from build123d import *

# Parameters (mm, degrees)
BOSS_EXTRUDE1_DEPTH = 19.05
SKETCH2_W           = 25.4
SKETCH2_H           = 6.35
BOSS_EXTRUDE2_DEPTH = 38.1
SKETCH3_R           = 6.35
CUT_EXTRUDE1_DEPTH  = 172.685024099
FILLET1_R           = 6.35
FILLET2_R           = 2.54
FILLET3_R           = 2.54


with BuildPart() as part:
    # Sketch1 → Boss-Extrude1 (new body)
    with BuildSketch(Plane(origin=(0, 0, 0), x_dir=(1, 0, 0), z_dir=(0, 1, 0))):
        with BuildLine():
            Line((-94.376875, 43.859194763), (4.54025, 27.568636708))
            ThreePointArc((4.54025, 27.568636708), (27.94, 0), (4.54025, -27.568636708))
            Line((4.54025, -27.568636708), (-94.376875, -43.859194763))
            ThreePointArc((-94.376875, -43.859194763), (-146.05, 0), (-94.376875, 43.859194763))
        make_face()
    extrude(amount=BOSS_EXTRUDE1_DEPTH)

    # Sketch2 → Boss-Extrude2 (add)
    with BuildSketch(Plane(origin=(0, 19.05, 0), x_dir=(1, 0, 0), z_dir=(0, 1, 0))):
        with Locations((-101.6, 22.225)):
            Rectangle(SKETCH2_W, SKETCH2_H)
        with Locations((-101.6, -22.225)):
            Rectangle(SKETCH2_W, SKETCH2_H)
    extrude(amount=BOSS_EXTRUDE2_DEPTH)

    # Sketch3 → Cut-Extrude1 (cut, through all)
    with BuildSketch(Plane.XY.offset(25.4)):
        with BuildLine():
            Line((-114.3, 57.15), (-114.3, 34.925))
            ThreePointArc((-114.3, 34.925), (-101.6, 47.625), (-88.9, 34.925))
            Line((-88.9, 34.925), (-88.9, 57.15))
            Line((-88.9, 57.15), (-114.3, 57.15))
        make_face()
        with Locations((-101.6, 34.925)):
            Circle(SKETCH3_R)
    extrude(amount=-CUT_EXTRUDE1_DEPTH, mode=Mode.SUBTRACT)

    # Fillet1
    fillet1_edges = [part.edges().sort_by_distance(p)[0] for p in [
        (27.94, 19.05, 0),
        (-44.9183125, 19.05, -35.713915735),
        (-146.05, 19.05, 0),
        (-44.9183125, 19.05, 35.713915735),
    ]]
    fillet(fillet1_edges, radius=FILLET1_R)

    # Fillet2
    fillet2_edges = [part.edges().sort_by_distance(p)[0] for p in [
        (-44.9183125, 0, -35.713915735),
        (27.94, 0, 0),
        (-44.9183125, 0, 35.713915735),
        (-146.05, 0, 0),
    ]]
    fillet(fillet2_edges, radius=FILLET2_R)

    # Fillet3
    fillet3_edges = [part.edges().sort_by_distance(p)[0] for p in [
        (-88.9, 26.9875, 25.4),
        (-114.3, 26.9875, 25.4),
        (-114.3, 26.9875, -25.4),
        (-88.9, 26.9875, -25.4),
        (-101.6, 47.625, -25.4),
        (-101.6, 47.625, 25.4),
    ]]
    fillet(fillet3_edges, radius=FILLET3_R)


solid = part.part
Can you work these out from the model? Positions are in its coordinate system, mm. A direction names the side the tool comes from. Coordinates: 2 decimals unless noted, no trailing zeros. Loops run counter-clockwise (first coordinate to the right, second up) from the corner with the lowest first, then second, coordinate; pieces in that order, holes last. Notation, with made-up numbers: M 9,-32 L 39,-32 A16 cw 39,-2 Z; hole C 13.5,-22.5 d7. An arc over 180 degrees is marked long. Return JSON: item names as keys, results as strings. Group by question number.
Item 1: Thinking about a two-plate mould opening in Z: for faces 1 (the flat face through (-102, 27, -19.05)), 2 (the cylindrical face through (-107.944, 35.204, 22.269)), 3 (the flat face through (-102, 26, -25.4)), 4 (the flat face through (-102, 27, 19.05)), which applies, released by +Z, released by -Z, zero draft, split by the parting line, or undercut?
Item 2: If I drill on L1, parallel to Y at x = -101.6, z = -21.5 (3 decimals); L2, parallel to Y at x = -67, z = -3.5; L3, parallel to X at y = 21.5, z = -20, over which ranges is the centre line in solid material (lowest first)? Write a range as from..to.
Item 3: On a 3-axis mill with a long thin cutter (end or side, diameter ignored), from which of +Z, -Z, +X, -X, +Y, -Y can I reach the whole of each face in a straight line? I mean faces 5 (the flat face through (-114.3, 27, 21)), 6 (the cylindrical face through (-101.88, 47.62, 20.98)), 7 (the flat face through (-88.9, 27, -21)), 8 (the flat face through (-45.611, 7.549, -35.828)), 9 (the flat face through (-102, 26, 25.4)). Say none if no direction works.
Item 4: Imagine slicing it at C-C (y = 5.5). Please give me the cut outline in (x, z).
Item 5: I'm going to push flat-ended pins straight in: pin 1 Ø3 at (y, z) = (24.5, -21.5) entering from +X; pin 2 Ø14.5 at (x, y) = (-101.6, 34.925) entering from +Z; pin 3 Ø10 at (x, z) = (-57, 27.5) entering from +Y. Where does each tip first touch, or does it pass through?
Item 6: Imagine slicing it at A-A (z = 0). Please give me the cut outline in (x, y), and give its area (3 significant figures).
Item 7: Imagine slicing it at B-B (x = -101.6). Give the number of separate pieces and of enclosed holes in the cut face, and give its area (3 significant figures).
Verdict:
{
 "1": {"face 1": "undercut", "face 2": "zero draft", "face 3": "released by -Z", "face 4": "undercut"},
 "2": {"L1": "y = 0..28.575, 41.275..47.625", "L2": "y = 0..19.05", "L3": "x = -114.3..-88.9"},
 "3": {"face 5": "+Z, -Z, -X, +Y", "face 6": "+Z, -Z, +Y", "face 7": "+Z, -Z, +X, +Y", "face 8": "-Z, +X, +Y, -Y", "face 9": "+Z, +X, -X, +Y"},
 "4": {"outline": "M -94.38,-43.86 L 4.54,-27.57 A27.94 ccw 4.54,27.57 L -94.38,43.86 A44.45 ccw long Z"},
 "5": {"pin 1": "stops at x = -88.9", "pin 2": "stops at z = 25.4", "pin 3": "stops at y = 19.05"},
 "6": {"outline": "M -146.05,2.54 A2.54 ccw -143.51,0 L 25.4,0 A2.54 ccw 27.94,2.54 L 27.94,12.7 A6.35 ccw 21.59,19.05 L -139.7,19.05 A6.35 ccw -146.05,12.7 Z", "area": "3,290 mm^2"},
 "7": {"separate pieces": "3", "enclosed holes": "0", "area": "1,870 mm^2"}
}
